Work out the finished part from the listing and answer in its coordinate system (mm). Face numbers are marked on the shaded views. A direction names the side the tool comes from. Give positions to 0.01 mm unless a question says otherwise; leave off trailing zeros. Order: outer loops, then holes, each group sorted by start corner. A loop starts at its lowest first (then second) coordinate and runs counter-clockwise, first axis right, second up. Notation, with made-up numbers: (-1.75, 49) -> (16.25, 49) arc R20 cw to (16.25, 63) -> close; hole circle Ø2 at (55, 9). An arc over 180 degrees is marked (long way). Use a Markdown table: item, result. Add a question column.
```python
from build123d import *

# Parameters (mm, degrees)
SKETCH1_W           = 110
SKETCH1_H           = 30
BOSS_EXTRUDE1_DEPTH = 5
SKETCH2_W           = 110
SKETCH2_H           = 25
BOSS_EXTRUDE2_DEPTH = 25
SKETCH6_R           = 3.429
CUT_EXTRUDE4_DEPTH  = 73.456883731
SKETCH7_W           = 40
SKETCH7_H           = 3
SKETCH7_W_2         = 20
SKETCH7_H_2         = 12
SKETCH7_W_3         = 22
CUT_EXTRUDE5_DEPTH  = 73.456883731
SKETCH8_W           = 110
SKETCH8_H           = 6.35
CUT_EXTRUDE6_DEPTH  = 73.456883731
FILLET1_R           = 10


with BuildPart() as part:
    # Sketch1 → Boss-Extrude1 (new body)
    with BuildSketch(Plane(origin=(0, 0, 0), x_dir=(1, 0, 0), z_dir=(0, 1, 0))):
        Rectangle(SKETCH1_W, SKETCH1_H)
    extrude(amount=BOSS_EXTRUDE1_DEPTH)

    # Sketch2 → Boss-Extrude2 (add)
    with BuildSketch(Plane.XY.offset(15)):
        with Locations((0, -7.5)):
            Rectangle(SKETCH2_W, SKETCH2_H)
    extrude(amount=BOSS_EXTRUDE2_DEPTH)

    # Sketch6 → Cut-Extrude4 (cut, through all)
    with BuildSketch(Plane(origin=(0, 5, 0), x_dir=(1, 0, 0), z_dir=(0, 1, 0))):
        with Locations(Location((-30, 0, 0), (0, 0, 270))):
            Circle(SKETCH6_R)
        with Locations(Location((30, 0, 0), (0, 0, 270))):
            Circle(SKETCH6_R)
    extrude(amount=-CUT_EXTRUDE4_DEPTH, mode=Mode.SUBTRACT)

    # Sketch7 → Cut-Extrude5 (cut, through all)
    with BuildSketch(Plane(origin=(0, 5, 0), x_dir=(1, 0, 0), z_dir=(0, 1, 0))):
        with Locations((0, -27.5)):
            Rectangle(SKETCH7_W, SKETCH7_H)
        with Locations((40, -27.5)):
            Rectangle(SKETCH7_W_2, SKETCH7_H_2)
        with Locations((-39, -27.5)):
            Rectangle(SKETCH7_W_3, SKETCH7_H)
    extrude(amount=-CUT_EXTRUDE5_DEPTH, mode=Mode.SUBTRACT)

    # Sketch8 → Cut-Extrude6 (cut, through all)
    with BuildSketch(Plane(origin=(0, 5, 0), x_dir=(1, 0, 0), z_dir=(0, 1, 0))):
        with Locations((0, 11.825)):
            Rectangle(SKETCH8_W, SKETCH8_H)
    extrude(amount=-CUT_EXTRUDE6_DEPTH, mode=Mode.SUBTRACT)

    # Fillet1
    fillet1_edges = [part.edges().sort_by_distance(p)[0] for p in [
        (-55, -7.5, 40),
        (55, -7.5, 40),
        (-55, 2.5, -8.65),
        (55, 2.5, -8.65),
    ]]
    fillet(fillet1_edges, radius=FILLET1_R)


solid = part.part
```
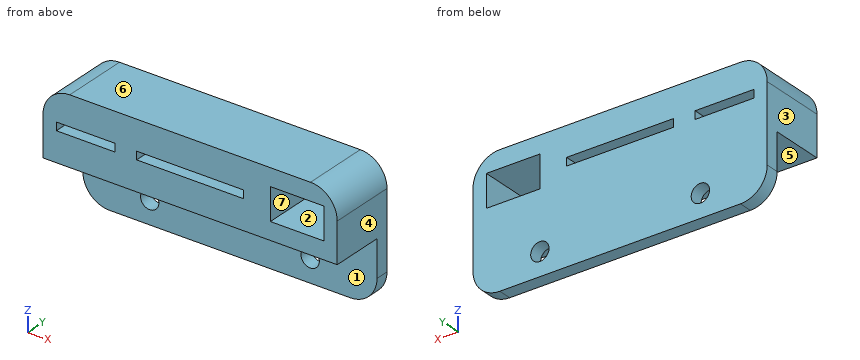
1) Determine the mould class of the marked faces 1, 2, 3 and 4 for opening direction X: released by +X, released by -X, zero draft, split by the parting line, or undercut.
2) Straight lines are drawn through the part: line 1 (Z direction, x = 17, y = -3.25); line 2 (X direction, y = 3.45, z = 0); line 3 (Z direction, x = 40.5, y = -7.5). For each, find the intervals that lie inside material, in ascending order.
3) The part is cut by section D-D, the plane z = 0. Determine the outline of the cut face in (x, y).
4) Flat-ended cylindrical pins translate along their axes: pin 1 (6 mm diameter, centred on x = 37, z = 24, fed in from +Y); pin 2 (11 mm diameter, centred on x = -30, z = 0, fed in from -Y). Find the tip coordinate at first contact, or state that the pin passes through.
5) The part is cut by section C-C, the plane y = -11.75. Determine the outline of the cut face in (x, z).
6) Which of the six approach directions +Z, -Z, +X, -X, +Y, -Y give full straight-line access (tool end or side, diameter ignored) to the marked faces 5, 6 and 7?
7) The part is cut by section B-B, the plane x = -30. Determine the outline of the cut face in (y, z), then the cut area to 3 significant figures.
8) The part is cut by section A-A, the plane x = -8. Determine the outline of the cut face in (y, z), then the cut area to 3 significant figures.
A:
| question | item | result |
|---|---|---|
| 1 | face 1 | zero draft |
| 1 | face 2 | undercut |
| 1 | face 3 | released by -X |
| 1 | face 4 | released by +X |
| 2 | line 1 | 15 to 26, 29 to 40 |
| 2 | line 2 | -54.91 to -33.43, -26.57 to 26.57, 33.43 to 54.91 |
| 2 | line 3 | 15 to 21.5, 33.5 to 40 |
| 3 | outline | (-54.91, 0) -> (-33.43, 0) -> (-33.43, 5) -> (-54.91, 5) -> close; (-26.57, 0) -> (26.57, 0) -> (26.57, 5) -> (-26.57, 5) -> close; (33.43, 0) -> (54.91, 0) -> (54.91, 5) -> (33.43, 5) -> close |
| 4 | pin 1 | y = 5 |
| 4 | pin 2 | y = 0 |
| 5 | outline | (-55, 15) -> (55, 15) -> (55, 30) arc R10 ccw to (45, 40) -> (-45, 40) arc R10 ccw to (-55, 30) -> close; hole (-50, 26) -> (-28, 26) -> (-28, 29) -> (-50, 29) -> close; hole (-20, 26) -> (20, 26) -> (20, 29) -> (-20, 29) -> close; hole (30, 21.5) -> (50, 21.5) -> (50, 33.5) -> (30, 33.5) -> close |
| 6 | face 5 | -Z, +X, -X, -Y |
| 6 | face 6 | +Z, +X, -X, +Y, -Y |
| 6 | face 7 | +Y, -Y |
| 7 | outline | (-20, 15) -> (0, 15) -> (0, 3.43) -> (5, 3.43) -> (5, 26) -> (-20, 26) -> close; (-20, 29) -> (5, 29) -> (5, 40) -> (-20, 40) -> close; (0, -8.65) -> (5, -8.65) -> (5, -3.43) -> (0, -3.43) -> close |
| 7 | area | 634 mm^2 |
| 8 | outline | (-20, 15) -> (0, 15) -> (0, -8.65) -> (5, -8.65) -> (5, 26) -> (-20, 26) -> close; (-20, 29) -> (5, 29) -> (5, 40) -> (-20, 40) -> close |
| 8 | area | 668 mm^2 |
